The listing builds one solid part. Answer for the finished solid, in the listing's coordinates (mm). Give positions to 0.01 mm unless a question says otherwise; leave off trailing zeros. Answer in a Markdown table with one row per item. Add a question column.
from build123d import *

# Parameters (mm, degrees)
SKETCH1_R           = 2.1
BOSS_EXTRUDE1_DEPTH = 180


with BuildPart() as part:
    # Sketch1 → Boss-Extrude1 (new body)
    with BuildSketch(Plane.XY):
        with BuildLine():
            Line((4.58, -10), (9.5, -10))
            ThreePointArc((9.5, -10), (9.853553391, -9.853553391), (10, -9.5))
            Line((10, -9.5), (10, -4.58))
            Line((10, -4.58), (8.545, -3.125))
            Line((8.545, -3.125), (8.2, -3.125))
            Line((8.2, -3.125), (8.2, -5.5))
            Line((8.2, -5.5), (6.560660172, -5.5))
            Line((6.560660172, -5.5), (3.9, -2.839339828))
            Line((3.9, -2.839339828), (3.9, -0.21))
            Line((3.9, -0.21), (3.69, 0))
            Line((3.69, 0), (3.9, 0.21))
            Line((3.9, 0.21), (3.9, 2.839339828))
            Line((3.9, 2.839339828), (6.560660172, 5.5))
            Line((6.560660172, 5.5), (8.2, 5.5))
            Line((8.2, 5.5), (8.2, 3.125))
            Line((8.2, 3.125), (8.545, 3.125))
            Line((8.545, 3.125), (10, 4.58))
            Line((10, 4.58), (10, 9.5))
            ThreePointArc((10, 9.5), (9.853553391, 9.853553391), (9.5, 10))
            Line((9.5, 10), (4.58, 10))
            Line((4.58, 10), (3.125, 8.545))
            Line((3.125, 8.545), (3.125, 8.2))
            Line((3.125, 8.2), (5.5, 8.2))
            Line((5.5, 8.2), (5.5, 6.560660172))
            Line((5.5, 6.560660172), (2.839339828, 3.9))
            Line((2.839339828, 3.9), (0.21, 3.9))
            Line((0.21, 3.9), (0, 3.69))
            Line((0, 3.69), (-0.21, 3.9))
            Line((-0.21, 3.9), (-2.839339828, 3.9))
            Line((-2.839339828, 3.9), (-5.5, 6.560660172))
            Line((-5.5, 6.560660172), (-5.5, 8.2))
            Line((-5.5, 8.2), (-3.125, 8.2))
            Line((-3.125, 8.2), (-3.125, 8.545))
            Line((-3.125, 8.545), (-4.58, 10))
            Line((-4.58, 10), (-9.5, 10))
            ThreePointArc((-9.5, 10), (-9.853553391, 9.853553391), (-10, 9.5))
            Line((-10, 9.5), (-10, 4.58))
            Line((-10, 4.58), (-8.545, 3.125))
            Line((-8.545, 3.125), (-8.2, 3.125))
            Line((-8.2, 3.125), (-8.2, 5.5))
            Line((-8.2, 5.5), (-6.560660172, 5.5))
            Line((-6.560660172, 5.5), (-3.9, 2.839339828))
            Line((-3.9, 2.839339828), (-3.9, 0.21))
            Line((-3.9, 0.21), (-3.69, 0))
            Line((-3.69, 0), (-3.9, -0.21))
            Line((-3.9, -0.21), (-3.9, -2.839339828))
            Line((-3.9, -2.839339828), (-6.560660172, -5.5))
            Line((-6.560660172, -5.5), (-8.2, -5.5))
            Line((-8.2, -5.5), (-8.2, -3.125))
            Line((-8.2, -3.125), (-8.545, -3.125))
            Line((-8.545, -3.125), (-10, -4.58))
            Line((-10, -4.58), (-10, -9.5))
            ThreePointArc((-10, -9.5), (-9.853553391, -9.853553391), (-9.5, -10))
            Line((-9.5, -10), (-4.58, -10))
            Line((-4.58, -10), (-3.125, -8.545))
            Line((-3.125, -8.545), (-3.125, -8.2))
            Line((-3.125, -8.2), (-5.5, -8.2))
            Line((-5.5, -8.2), (-5.5, -6.560660172))
            Line((-5.5, -6.560660172), (-2.839339828, -3.9))
            Line((-2.839339828, -3.9), (-0.21, -3.9))
            Line((-0.21, -3.9), (0, -3.69))
            Line((0, -3.69), (0.21, -3.9))
            Line((0.21, -3.9), (2.839339828, -3.9))
            Line((2.839339828, -3.9), (5.5, -6.560660172))
            Line((5.5, -6.560660172), (5.5, -8.2))
            Line((5.5, -8.2), (3.125, -8.2))
            Line((3.125, -8.2), (3.125, -8.545))
            Line((3.125, -8.545), (4.58, -10))
        make_face()
        with Locations(Location((0, 0, 0), (0, 0, 180))):
            Circle(SKETCH1_R, mode=Mode.SUBTRACT)
    extrude(amount=BOSS_EXTRUDE1_DEPTH)


solid = part.part
1. The mould has two halves that part along Y. Classify faces 1 (the face through (-2.003, -0.631, 88.74)), 2 (the face through (7, 10, 89)), 3 (the face through (-7, -10, 89)): +Y half, -Y half, draft (parallel to the pull), parting line (faces both ways), or undercut.
2. Given pin 1 Ø0.8 at (y, z) = (2, 45.5) entering from +X; pin 2 Ø5 at (x, y) = (0, 0) entering from -Z; pin 3 Ø1 at (y, z) = (3.5, 75) entering from +X; pin 4 Ø3 at (y, z) = (1, 77.5) entering from -X, each flat-ended and moving along its own axis, determine where each tip first touches the part or whether it passes through.
3. Straight lines are drawn through the part: L1, parallel to Y at x = -7.5, z = 33; L2, parallel to Y at x = 0, z = 133. For each, find the intervals that lie inside material, in ascending order. Write a range as [from, to].
Geometry check:
| question | item | result |
|---|---|---|
| 1 | face 1 | undercut |
| 1 | face 2 | +Y half |
| 1 | face 3 | -Y half |
| 2 | pin 1 | x = 3.9 |
| 2 | pin 2 | z = 0 |
| 2 | pin 3 | x = 9.42 |
| 2 | pin 4 | x = -3.9 |
| 3 | L1 | [-10, -5.5], [5.5, 10] |
| 3 | L2 | [-3.69, -2.1], [2.1, 3.69] |
